Part model, mm, in its own coordinate system. A direction names the side the tool comes from. Coordinates: 2 decimals unless noted, no trailing zeros. Loops run counter-clockwise (first coordinate to the right, second up) from the corner with the lowest first, then second, coordinate; pieces in that order, holes last. Notation, with made-up numbers: M 70.25,-14.75 L 89.25,-14.75 A26 cw 89.25,0.25 Z; hole C -9.75,-37 d8. An arc over 180 degrees is marked long. Answer as CSV lines item,"result". Start each with the question number.
from build123d import *

# Parameters (mm, degrees)
F0_W     = 2.54
F0_H     = 0.976924
F1_DEPTH = 45.72
F2_R     = 0.499245
F3_DEPTH = 25.4
F4_R     = 0.551082
F5_DEPTH = 50.8


with BuildPart() as f1:
    # F0 (on Front) → F1 (new body)
    with BuildSketch(Plane.XZ):
        Rectangle(F0_W, F0_H)
    extrude(amount=F1_DEPTH)

    # F2 (on face) → F3 (cut)
    with BuildSketch(Plane.XY.offset(0.488462)):
        with Locations((0, -44.554785)):
            Circle(F2_R)
    extrude(amount=-F3_DEPTH, mode=Mode.SUBTRACT)

    # F4 (on Top) → F5 (cut)
    with BuildSketch(Plane.XY):
        with Locations((0, -1.580954)):
            Circle(F4_R)
    extrude(amount=-F5_DEPTH, mode=Mode.SUBTRACT)


solid = f1.part
Q1. Tool access for faces 5 (the face through (0, -1.6, 0)), 6 (the face through (-1.27, -23, 0)): list every direction of +Z, -Z, +X, -X, +Y, -Y with a clear straight run to the whole face (end or side of a thin tool).
Q2. Two-plate mould, pull along Y, no slides. Class faces 1 (the face through (0, 0, 0)), 2 (the face through (0, -23, 0.488)), 3 (the face through (0, -45.72, 0)), 4 (the face through (-0.06, -44.06, 0.01)): +Y half, -Y half, draft (parallel to the pull), parting line (faces both ways), or undercut.
Q3. Slice it at A-A, the plane x = 0. Write the cut outline in (y, z), and give its area (3 significant figures).
Q4. Wall check: L1, parallel to Y at x = 0, z = -0.2; L2, parallel to Y at x = -0.1, z = -0.15; L3, parallel to Y at x = 0, z = 0.35. Give the ranges that are in metal, low to high.
Solved:
1,face 5,"-Z"
1,face 6,"+Z, -Z, -X, +Y, -Y"
2,face 1,"+Y half"
2,face 2,"draft"
2,face 3,"-Y half"
2,face 4,"undercut"
3,outline,"M -45.72,-0.49 L -45.05,-0.49 L -45.05,0.49 L -45.72,0.49 Z; M -44.06,-0.49 L -2.13,-0.49 L -2.13,0 L -1.03,0 L -1.03,-0.49 L 0,-0.49 L 0,0.49 L -44.06,0.49 Z"
3,area,"43.2 mm2"
4,L1,"y = -45.72 to -45.05, -44.06 to -2.13, -1.03 to 0"
4,L2,"y = -45.72 to -45.04, -44.07 to -2.12, -1.04 to 0"
4,L3,"y = -45.72 to -45.05, -44.06 to 0"
